Model file for the job. Use its own axes, mm. A direction names the side the tool comes from. Give positions to 0.01 mm unless a question says otherwise; leave off trailing zeros. Write each loop counter-clockwise with the first axis right and the second up, starting at its lowest first coordinate (ties: lowest second). Pieces come first, ordered by that corner, then holes.
Autodesk Inventor part; units mm, degrees
ref_plane "YZ Plane" through (0, 0, 0) normal (1, 0, 0) x (0, 1, 0)
ref_plane "XZ Plane" through (0, 0, 0) normal (0, 1, 0) x (-1, 0, 0)
ref_plane "XY Plane" through (0, 0, 0) normal (0, 0, 1) x (1, 0, 0)
sketch "Sketch1" plane through (0, 0, 0) normal (0, 0, 1) x (1, 0, 0)
  circle A0 centre (152.0025, 356.0058) radius 5
  line L0 (28.751, 0) -> (220.0553, 108.6482)
  line L1 (220.0553, 108.6482) -> (233.0937, 120.8954)
  line L2 (233.0937, 120.8954) -> (159.1798, 368.1207)
  line L3 (159.1798, 368.1207) -> (141.7433, 362.9081)
  line L4 (141.7433, 362.9081) -> (196.9837, 143.9375)
  line L5 (196.9837, 143.9375) -> (-13.7687, 24.2435)
  line L6 (0, 0) -> (-13.7687, 24.2435)
  line L7 (0, 0) -> (28.751, 0)
  dimension "CHAMFER" = 28.751
  dimension "d1" = 60.406
  dimension "d2" = 29.594
  dimension "ARM_L" = 220.004
  dimension "ARM_L2" = 242.37
  dimension "ARM_VER_L" = 258.038
  dimension "ARM_VER_L2" = 225.831
  dimension "ARM_W2" = 18.199
  dimension "ARM_W" = 42.162
  dimension "PIN_HOLE" = 10
  dimension "d10" = 233.0937
  dimension "d11" = 120.8954
  dimension "d12" = 24.2435
  dimension "d13" = 13.7687
  dimension "d14" = 196.9837
  dimension "d15" = 220.0553
  dimension "d16" = 159.1798
  dimension "d17" = 152.0025
  dimension "d18" = 356.0058
extrude "Extrusion1" add sketch "Sketch1" along normal mid plane 23
sketch "Sketch2" plane through (0, 0, -11.5) normal (0, 0, -1) x (-1, 0, 0)
  line L0 (-7.9703, 36.5899) -> (13.7687, 24.2435)
  line L1 (13.7687, 24.2435) -> (-0.054, -0.0951)
  line L2 (0, 0) -> (-0.054, -0.0951)
  line L3 (0, 0) -> (-28.751, 0)
  line L4 (-7.9703, 36.5899) -> (-28.751, 0)
  line L5 (0, 0) -> (13.7687, 24.2435)
  line L6 (13.7687, 24.2435) -> (-196.9837, 143.9375)
  line L7 (-28.751, 0) -> (0, 0)
  point P0 (226.376, 276)
extrude "Extrusion2" add sketch "Sketch2" along normal blind 274
sketch "Sketch3" plane through (196.9837, 143.9375, 11.5) normal (-0.4938, 0.8695, 0) x (0.8695, 0.4938, 0)
  line L0 (-242.3701, 0) -> (-217.3697, 0)
  line L1 (-242.3701, 0) -> (-241.6771, 0)
  line L2 (-241.6771, 0) -> (-241.6771, 63.016)
  line L3 (-241.6771, 63.016) -> (-242.3701, 63.016)
  line L4 (-242.3701, 63.016) -> (-242.3701, 0)
  point P0 (-242.3701, 11.5)
  point P1 (-241.6771, 0)
  dimension "d23" = 63.016
  dimension "d24" = 0.693
extrude "Extrusion3" cut sketch "Sketch3" against normal blind 274
properties part number "grip - C2-1"
1. Which spindle directions (+Z, -Z, +X, -X, +Y, -Y) get a long thin tool onto all of the face, cutting with end or side? Do faces 4 (the flat face through (-6.6, 12.3, -51.516)), 5 (the flat face through (18.215, 18.551, -146.582)), 6 (the flat face through (168.977, 254.956, -0.161)). Say none if no direction does.
Calculated:
face 4: +Z, -X, -Y
face 5: -Z, +X, +Y
face 6: +Z, -Z, -X
2. Slice it at A-A, the plane z = -99. Write the cut outline in (x, y).
Calculated:
outline: (-13.77, 24.24) - (0, 0) - (28.75, 0) - (7.97, 36.59) - close
3. Probe probe 1 along Z at (x, y) = (78, 66.5); probe 2 along X at (y, z) = (22.5, -210.5); probe 3 along X at (y, z) = (30.5, -232). List the from-to ranges inside material, lowest first.
Calculated:
probe 1: z = -11.5 to 11.5
probe 2: x = -12.78 to 15.97
probe 3: x = -2.75 to 11.43
4. Slice it at B-B, the plane x = 93. Write the cut outline in (y, z).
Calculated:
outline: (36.49, -11.5) - (84.88, -11.5) - (84.88, 11.5) - (36.49, 11.5) - close
5. Pin check, flat tip, straight feed: P1, Ø2, axis at x = 101.5, y = 74, coming from the -Z side. Stop position of the tip, or through.
Calculated:
P1: stops at z = -11.5
6. Pull direction X, two halves, no side cores. Call faces 1 (the cylindrical face through (154.31, 360.44, -0.16)), 2 (the flat face through (-6.98, 12.29, -166.87)), 3 (the flat face through (8, 14, -285.5)): +X half, -X half, draft (parallel to the pull), parting line (faces both ways), or undercut.
Calculated:
face 1: undercut
face 2: -X half
face 3: draft
